Autodesk Inventor part; units mm, degrees
ref_plane "YZ Plane" through (0, 0, 0) normal (1, 0, 0) x (0, 1, 0)
ref_plane "XZ Plane" through (0, 0, 0) normal (0, 1, 0) x (-1, 0, 0)
ref_plane "XY Plane" through (0, 0, 0) normal (0, 0, 1) x (1, 0, 0)
sketch "Sketch1" plane through (0, 0, 0) normal (0, 1, 0) x (-1, 0, 0)
  line L0 (-70, 85) -> (70, 85)
  line L1 (70, 85) -> (70, -85)
  line L2 (70, -85) -> (-70, -85)
  line L3 (-70, -85) -> (-70, 85)
  line L4 (-70, 85) -> (70, -85) construction
  line L5 (70, 85) -> (-70, -85) construction
  line L6 (98, 0) -> (-98, 0)
  line L7 (70, -85) -> (50, -85)
  line L8 (50, -85) -> (50, -30)
  line L9 (50, -30) -> (70, -30)
  line L10 (70, -30) -> (70, -85)
  line L11 (-70, -85) -> (-50, -85)
  line L12 (-50, -85) -> (-50, -30)
  line L13 (-50, -30) -> (-70, -30)
  line L14 (-70, -30) -> (-70, -85)
  point P0 (0, 0)
  dimension "d0" = 140
  dimension "d1" = 170
  dimension "d35" = 20
  dimension "d36" = 55
  dimension "d37" = 20
  dimension "d38" = 55
extrude "Extrusion1" add sketch "Sketch1" along normal blind 4 contours L0 L1 L6 L3 | L6 L1 L9 L8 L2 L12 L13 L3
fillet "Fillet1" radius 15 2 edges at (-70, 2, 85) (70, 2, 85)
fillet "Fillet2" radius 15 2 edges at (-50, 2, -85) (50, 2, -85)
sketch "Sketch2" plane through (0, 4, 0) normal (0, 1, 0) x (1, 0, 0)
  line L0 (-70, 30) -> (-70, -70)
  arc A0 (-70, -70) -> (-55, -85) centre (-55, -70) ccw
  line L1 (-55, -85) -> (55, -85)
  arc A1 (55, -85) -> (70, -70) centre (55, -70) ccw
  line L2 (70, -70) -> (70, 30)
  line L3 (35, 85) -> (-35, 85)
  line L4 (70, 30) -> (50, 30)
  line L5 (50, 30) -> (50, 70)
  line L6 (-50, 70) -> (-50, 30)
  line L7 (-50, 30) -> (-70, 30)
  arc A2 (50, 70) -> (35, 85) centre (35, 70) ccw
  arc A3 (-35, 85) -> (-50, 70) centre (-35, 70) ccw
  point P0 (0, 0)
  point P1 (-4.3272, -2.2983)
hole "Hole1" at (55, 4, 70) at (-55, 4, 70) at (35, 4, -70) at (-35, 4, -70) direction (0, -1, 0) diameter 10 depth 4
sketch "Sketch3" plane through (0, 4, 0) normal (0, 1, 0) x (1, 0, 0)
  line L0 (22.8472, -55) -> (-47.1528, -55)
  line L1 (-47.1528, -55) -> (-47.1528, 27)
  line L2 (-47.1528, 27) -> (22.8472, 27)
  line L3 (22.8472, 27) -> (22.8472, -55)
  line L4 (22.8472, -55) -> (-47.1528, 27) construction
  line L5 (-47.1528, -55) -> (22.8472, 27) construction
  line L6 (-55, -85) -> (55, -85)
  point P0 (0, 0)
  point P1 (-12.1528, -14)
  dimension "d12" = 70
  dimension "d13" = 82
  dimension "d34" = 30
fillet "Fillet3" radius 5 4 edges at (-50, 2, -30) (-70, 2, -30) (70, 2, -30) (50, 2, -30)
sketch "Sketch5" plane through (0, 4, 0) normal (0, 1, 0) x (1, 0, 0)
  line L0 (-55, 12.5998) -> (-25, 12.5998)
  line L1 (-25, 12.5998) -> (-25, -27.4002)
  line L2 (-25, -27.4002) -> (-55, -27.4002)
  line L3 (-55, -27.4002) -> (-55, 12.5998)
  line L4 (0, -27.4002) -> (0, 4.9411)
  line L5 (-24, -76.5868) -> (24, -76.5868)
  line L6 (26, -74.5868) -> (26, -49.5868)
  line L7 (24, -47.5868) -> (-24, -47.5868)
  line L8 (-26, -49.5868) -> (-26, -74.5868)
  arc A0 (24, -76.5868) -> (26, -74.5868) centre (24, -74.5868) ccw
  arc A1 (-24, -47.5868) -> (-26, -49.5868) centre (-24, -49.5868) ccw
  arc A2 (26, -49.5868) -> (24, -47.5868) centre (24, -49.5868) ccw
  arc A3 (-26, -74.5868) -> (-24, -76.5868) centre (-24, -74.5868) ccw
  circle A4 centre (24, -74.5868) radius 3
  circle A5 centre (24, -49.5868) radius 3
  circle A6 centre (-24, -49.5868) radius 3
  circle A7 centre (-24, -74.5868) radius 3
  line L9 (-22, -76.5868) -> (19, -76.5868)
  line L10 (19, -76.5868) -> (19, -72.5868)
  line L11 (19, -72.5868) -> (-22, -72.5868)
  line L12 (-22, -72.5868) -> (-22, -76.5868)
  line L13 (26, -62.0868) -> (21, -62.0868)
  line L14 (19, -47.5868) -> (19, -51.5868)
  line L15 (19, -51.5868) -> (-22, -51.5868)
  line L16 (-22, -51.5868) -> (-22, -47.5868)
  line L17 (55, 12.5998) -> (25, 12.5998)
  line L18 (25, 12.5998) -> (25, -27.4002)
  line L19 (25, -27.4002) -> (55, -27.4002)
  line L20 (5.6733, -33.7631) -> (-15.8267, -33.7631)
  line L21 (-17.8267, -31.7631) -> (-17.8267, -18.2631)
  line L22 (-17.8267, -18.2631) -> (7.6733, -18.2631)
  line L23 (7.6733, -18.2631) -> (7.6733, -31.7631)
  arc A8 (-17.8267, -31.7631) -> (-15.8267, -33.7631) centre (-15.8267, -31.7631) ccw
  arc A9 (-17.8267, -31.7631) -> (-15.8267, -33.7631) centre (-15.8267, -31.7631) ccw
  arc A10 (5.6733, -33.7631) -> (7.6733, -31.7631) centre (5.6733, -31.7631) ccw
  circle A11 centre (-15.8267, -31.7631) radius 2.5
  circle A12 centre (5.6733, -31.7631) radius 2.5
  line L24 (-17.8267, -18.2631) -> (7.6733, -18.2631)
  line L25 (7.6733, -18.2631) -> (7.6733, -21.2631)
  line L26 (7.6733, -21.2631) -> (-17.8267, -21.2631)
  line L27 (-17.8267, -21.2631) -> (-17.8267, -18.2631)
  line L28 (-17.8267, -18.2631) -> (7.6733, -18.2631)
  line L29 (7.6733, -18.2631) -> (7.6733, -17.2631)
  line L30 (7.6733, -17.2631) -> (-17.8267, -17.2631)
  line L31 (-17.8267, -17.2631) -> (-17.8267, -18.2631)
  point P0 (0, 0)
  point P1 (26, -47.5868)
  point P2 (26, -76.5868)
  point P3 (-26, -47.5868)
  point P4 (-17.8267, -33.7631)
  point P5 (-21.7639, -47.5868)
  point P6 (-21.7639, -51.5868)
  point P7 (-21.7639, -72.5868)
  point P8 (-21.7639, -76.5868)
  point P9 (19, -76.5868)
  dimension "d41" = 30
  dimension "d42" = 40
  dimension "d43" = 52
  dimension "d44" = 29
  dimension "d45" = 2
  dimension "d46" = 6
  dimension "d47" = 6
  dimension "d48" = 6
  dimension "d49" = 6
  dimension "d50" = 4
  dimension "d51" = 41
  dimension "d52" = 7
  dimension "d53" = 25.5
  dimension "d54" = 15.5
  dimension "d55" = 2
  dimension "d56" = 5
  dimension "d57" = 5
  dimension "d62" = 3
  dimension "d63" = 1
extrude "Extrusion3" cut sketch "Sketch5" against normal up to next contours L26 L21 L22 L4 | L4 L22 L23 L26 | L22 L31 L30 L4 | L4 L30 L29 L22 | A12 L20 A10 L23 | L23 A10 L20 A12 | A11 L20 A8 L21 | L21 A8 L20 A11 | A3 L8 A7 L11 L12 L5 | L5 A7 L8 A3 | L12 L11 A7 L5 | A7 L11 L10 L5 | A6 L7 A1 L8 | L8 A1 L7 L16 L15 A6 | A4 L6 A0 L5 | L5 A0 L6 A4 | A6 L15 L16 L7 | L7 L14 L15 A6 | A5 L6 A2 L7 | L7 A2 L6 A5
properties part number "Base2" material "PLA"
Source: CAD feature listing. Evaluate the final solid. Frame: model axes, mm. A direction names the side the tool comes from. Coordinates: 2 decimals unless noted, no trailing zeros. Loops run counter-clockwise (first coordinate to the right, second up) from the corner with the lowest first, then second, coordinate; pieces in that order, holes last. Notation, with made-up numbers: M 18.25,-14.75 L 65.25,-14.75 A9 ccw 65.25,-8.75 Z; hole C 61,55 d5. An arc over 180 degrees is marked long. Use a Markdown table: item, result. Add a question column.
Q1. Draft query along Z for faces 4 (the flat face through (0, 2, -85)), 5 (the cylindrical face through (-18.324, 2.028, 31.653)), 6 (the cylindrical face through (23.609, 2.028, 71.612)), 7 (the flat face through (-50, 2, -53)). Return one class per face: pulls with the +Z half, pulls with the -Z half, needs draft (parallel to the pull), parting line crosses it, or undercut.
Q2. First-contact query: pin 1 (8 mm diameter, centred on x = -24, z = 74.59, fed in from -Y); pin 2 (1.2 mm diameter, centred on y = 1.5, z = 74, fed in from -X); pin 3 (4 mm diameter, centred on x = 5.67, z = 31.76, fed in from -Y); pin 4 (1.2 mm diameter, centred on x = -60.5, y = 1.5, fed in from -Z). Flat tips, straight axial feed; report the tip coordinate or a pass-through.
Q3. Section query D-D, the plane x = -47. Return loops of the section in (y, z).
Q4. Material intervals for L1, parallel to X at y = 2.85, z = -70; L2, parallel to Z at x = 1, y = 1.5; L3, parallel to Z at x = 24, y = 2.55, sorted ascending.
Q5. Section query C-C, the plane z = -58. Return loops of the section in (x, y).
Q6. Access query for faces 1 (the flat face through (-60, 2, -30)), 2 (the cylindrical face through (69, 2, -28)), 3 (the flat face through (-17.827, 2, 19)). Directions: +Z, -Z, +X, -X, +Y, -Y. A direction counts if a zero-diameter tool reaches every point of the face in a straight line with its end or side. Return the directions, or none.
Q7. Section query A-A, the plane x = -24. Return loops of the section in (y, z), and give its area (3 significant figures).
Q8. Section query B-B, the plane y = 3.1. State how many separate pieces and enclosed holes the cut face has, and give its area (3 significant figures).
Result:
| question | item | result |
|---|---|---|
| 1 | face 4 | pulls with the -Z half |
| 1 | face 5 | undercut |
| 1 | face 6 | undercut |
| 1 | face 7 | needs draft |
| 2 | pin 1 | stops at y = 0 |
| 2 | pin 2 | stops at x = -69.61 |
| 2 | pin 3 | passes through |
| 2 | pin 4 | stops at z = -30 |
| 3 | outline | M 0,-79 L 4,-79 L 4,85 L 0,85 Z |
| 4 | L1 | x = -50 to -40, -30 to 30, 40 to 50 |
| 4 | L2 | z = -85 to 17.26, 21.26 to 47.59, 51.59 to 72.59, 76.59 to 85 |
| 4 | L3 | z = -85 to 46.59, 52.59 to 71.59, 77.59 to 85 |
| 5 | outline | M -50,0 L 50,0 L 50,4 L -50,4 Z |
| 6 | face 1 | -Z, -X, +Y, -Y |
| 6 | face 2 | -Z, +X, +Y, -Y |
| 6 | face 3 | +Y, -Y |
| 7 | outline | M 0,-85 L 4,-85 L 4,46.59 L 0,46.59 Z; M 0,52.59 L 4,52.59 L 4,71.59 L 0,71.59 Z; M 0,77.59 L 4,77.59 L 4,85 L 0,85 Z |
| 7 | area | 632 mm2 |
| 8 | separate pieces | 1 |
| 8 | enclosed holes | 11 |
| 8 | area | 20,500 mm2 |
